For this review, take the finished solid that the model builds, in its own axes (mm). Face numbers are marked on the shaded views. A direction names the side the tool comes from. Give positions to 0.01 mm unless a question says otherwise; leave off trailing zeros. Write each loop counter-clockwise with the first axis right and the second up, starting at its lowest first coordinate (ties: lowest second). Pieces come first, ordered by that corner, then holes. Notation, with made-up numbers: (-5.5, 1.5) -> (33.5, 1.5) arc R15 cw to (33.5, 21.5) -> close; hole circle Ø4 at (63.25, 8.5). An arc over 180 degrees is marked (long way). Write item = value, one per line.
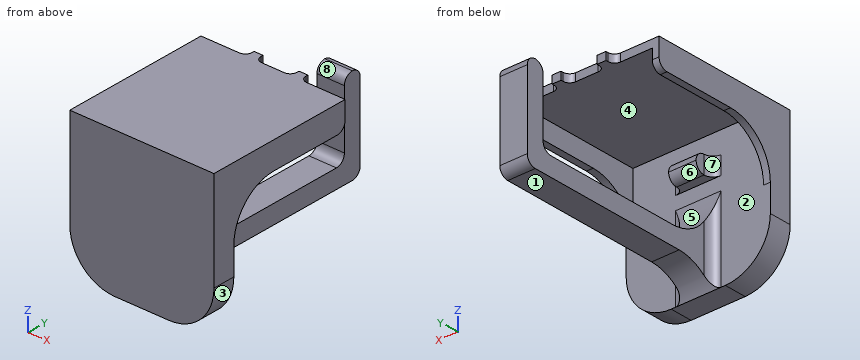
```python
from build123d import *

# Parameters (mm, degrees)
SKETCH1_W           = 32
SKETCH1_H           = 32
BOSS_EXTRUDE1_DEPTH = 5
BOSS_EXTRUDE5_DEPTH = 28
SKETCH6_W           = 6.1
SKETCH6_H           = 4.005404858
CUT_EXTRUDE2_DEPTH  = 24
SKETCH7_W           = 1.973672473
SKETCH7_H           = 2
BOSS_EXTRUDE6_DEPTH = 1.742972258
FILLET1_R           = 1.5
SKETCH8_W           = 6.1
SKETCH8_H           = 4.149014421
BOSS_EXTRUDE7_DEPTH = 42.5
SKETCH9_W           = 6.1
SKETCH9_H           = 3.972443091
BOSS_EXTRUDE8_DEPTH = 16.930897648
SKETCH10_W          = 6.1
SKETCH10_H          = 3.972443091
BOSS_EXTRUDE9_DEPTH = 4.149014421
FILLET3_R           = 2
FILLET5_R           = 10
FILLET6_R           = 2
FILLET7_R           = 10


with BuildPart() as part:
    # Sketch1 → Boss-Extrude1 (new body)
    with BuildSketch(Plane(origin=(0, 0, 0), x_dir=(1, 0, 0), z_dir=(0, 1, 0))):
        Rectangle(SKETCH1_W, SKETCH1_H)
    extrude(amount=BOSS_EXTRUDE1_DEPTH)

    # Sketch2 → Boss-Extrude5 (add)
    with BuildSketch(Plane(origin=(0, 5, 0), x_dir=(1, 0, 0), z_dir=(0, 1, 0))):
        Polygon((3.05, -5.451622884), (-3.05, -5.451622884), (-3.05, -9.457027742), (0, -9.457027742), (3.05, -9.457027742), align=None)
        Polygon((-14.5, -16), (0, -16), (14.5, -16), (16, -16), (16, -10), (14.5, -10), (14.5, -14.257027742), (0, -14.257027742), (-14.5, -14.257027742), (-14.5, -10), (-16, -10), (-16, -16), align=None)
    extrude(amount=BOSS_EXTRUDE5_DEPTH)

    # Sketch6 → Cut-Extrude2 (cut)
    with BuildSketch(Plane(origin=(0, 33, 0), x_dir=(1, 0, 0), z_dir=(0, 1, 0))):
        with Locations((0, -7.454325313)):
            Rectangle(SKETCH6_W, SKETCH6_H)
    extrude(amount=-CUT_EXTRUDE2_DEPTH, mode=Mode.SUBTRACT)

    # Sketch7 → Boss-Extrude6 (add)
    with BuildSketch(Plane.XY.offset(16)):
        with Locations((-4.986836237, 34)):
            Rectangle(SKETCH7_W, SKETCH7_H)
        with Locations((4.986836237, 34)):
            Rectangle(SKETCH7_W, SKETCH7_H)
    extrude(amount=-BOSS_EXTRUDE6_DEPTH)

    # Fillet1
    fillet1_edges = [part.edges().sort_by_distance(p)[0] for p in [
        (-5.973672473, 33, 15.128513871),
        (-4, 33, 15.128513871),
        (5.973672473, 33, 15.128513871),
        (4, 33, 15.128513871),
    ]]
    fillet(fillet1_edges, radius=FILLET1_R)

    # Sketch8 → Boss-Extrude7 (add)
    with BuildSketch(Plane(origin=(0, 5, 0), x_dir=(1, 0, 0), z_dir=(0, 1, 0))):
        with Locations((0, 9.548377117)):
            Rectangle(SKETCH8_W, SKETCH8_H)
    extrude(amount=BOSS_EXTRUDE7_DEPTH)



with BuildPart() as body_2:
    # Sketch9 → Boss-Extrude8 (new body)
    with BuildSketch(Plane.XY.offset(-7.473869906)):
        with Locations((0, 49.486221546)):
            Rectangle(SKETCH9_W, SKETCH9_H)
    extrude(amount=BOSS_EXTRUDE8_DEPTH)


with BuildPart() as part_1:
    add(part.part)

    add(body_2.part)  # Boss-Extrude9 merges body 2
    # Sketch10 → Boss-Extrude9 (add)
    with BuildSketch(Plane(origin=(0, 0, -7.473869906), x_dir=(-1, 0, 0), z_dir=(0, 0, -1))):
        with Locations((0, 49.486221546)):
            Rectangle(SKETCH10_W, SKETCH10_H)
    extrude(amount=BOSS_EXTRUDE9_DEPTH)

    # Fillet3
    # the kernel refuses this fillet: 2 mm, written as the material it adds along each edge
    with BuildSketch(Plane(origin=(3.05, 47.5, -7.473869906), x_dir=(0, 0, 1), z_dir=(-1, 0, 0))) as fillet3_piece_1:
        with BuildLine():
            CenterArc((FILLET3_R, -FILLET3_R), FILLET3_R, 90, 90)
            Line((0, -FILLET3_R), (0, 0))
            Line((0, 0), (FILLET3_R, 0))
        make_face()
    extrude(amount=6.1)
    # the kernel refuses this fillet: 2 mm, written as the material it takes off along each edge
    with BuildSketch(Plane(origin=(8.05, 51.472443091, -11.622884327), x_dir=(0, -1, 0), z_dir=(-1, 0, 0)), Plane(origin=(-8.05, 51.472443091, 9.457027742), x_dir=(0, -1, 0), z_dir=(1, 0, 0))) as fillet3_2_piece_1:
        with BuildLine():
            CenterArc((FILLET3_R, FILLET3_R), FILLET3_R, 180, 90)
            Line((0, FILLET3_R), (0, 0))
            Line((0, 0), (FILLET3_R, 0))
        make_face()
    extrude(amount=16.1, mode=Mode.SUBTRACT)
    with BuildSketch(Plane(origin=(8.05, 47.5, 9.457027742), x_dir=(0, 0, -1), z_dir=(-1, 0, 0)), Plane(origin=(-8.05, 9, 5.451622884), x_dir=(0, -1, 0), z_dir=(1, 0, 0)), Plane(origin=(8.05, 9, 9.457027742), x_dir=(0, -1, 0), z_dir=(-1, 0, 0))) as fillet3_2_piece_2:
        with BuildLine():
            CenterArc((FILLET3_R, -FILLET3_R), FILLET3_R, 90, 90)
            Line((0, -FILLET3_R), (0, 0))
            Line((0, 0), (FILLET3_R, 0))
        make_face()
    extrude(amount=16.1, mode=Mode.SUBTRACT)
    with BuildSketch(Plane(origin=(21, 33, 10), x_dir=(0, 0, 1), z_dir=(-1, 0, 0)), Plane(origin=(-9.5, 33, 10), x_dir=(0, 0, 1), z_dir=(-1, 0, 0))) as fillet3_2_piece_3:
        with BuildLine():
            CenterArc((FILLET3_R, -FILLET3_R), FILLET3_R, 90, 90)
            Line((0, -FILLET3_R), (0, 0))
            Line((0, 0), (FILLET3_R, 0))
        make_face()
    extrude(amount=11.5, mode=Mode.SUBTRACT)

    # Fillet5
    # the kernel refuses this fillet: 10 mm, written as the material it adds along each edge
    with BuildSketch(Plane(origin=(-3.05, 5, -7.473869906), x_dir=(0, 1, 0), z_dir=(1, 0, 0))) as fillet5_piece_1:
        with BuildLine():
            CenterArc((FILLET5_R, FILLET5_R), FILLET5_R, 180, 90)
            Line((0, FILLET5_R), (-FILLET5_R * 0.02, FILLET5_R))
            Line((-FILLET5_R * 0.02, FILLET5_R), (-FILLET5_R * 0.02, -FILLET5_R * 0.02))
            Line((-FILLET5_R * 0.02, -FILLET5_R * 0.02), (FILLET5_R, -FILLET5_R * 0.02))
            Line((FILLET5_R, -FILLET5_R * 0.02), (FILLET5_R, 0))
        make_face()
    extrude(amount=6.1)
    with BuildSketch(Plane(origin=(3.05, 5, -11.622884327), x_dir=(0, 0, -1), z_dir=(-1, 0, 0))) as fillet5_piece_2:
        with BuildLine():
            CenterArc((10, -8.26941182), FILLET5_R, 124.214206314, 55.785793686)
            Line((0, -8.26941182), (-0.2, -8.26941182))
            Line((-0.2, -8.26941182), (-0.2, 0))
            Line((-0.2, 0), (0, 0.2))
            ThreePointArc((0, 0.2), (2.188557837, 0.2), (4.264657987, 0.165388236))
            Line((4.264657987, 0.165388236), (4.377115673, 0))
        make_face()
    extrude(amount=6.1)
    with BuildSketch(Plane(origin=(-14.5, 5, 10), x_dir=(0, 0, -1), z_dir=(-1, 0, 0)), Plane(origin=(16, 5, 10), x_dir=(0, 0, -1), z_dir=(-1, 0, 0))) as fillet5_piece_3:
        with BuildLine():
            CenterArc((FILLET5_R, -FILLET5_R), FILLET5_R, 90, 90)
            Line((0, -FILLET5_R), (-FILLET5_R * 0.02, -FILLET5_R))
            Line((-FILLET5_R * 0.02, -FILLET5_R), (-FILLET5_R * 0.02, FILLET5_R * 0.02))
            Line((-FILLET5_R * 0.02, FILLET5_R * 0.02), (FILLET5_R, FILLET5_R * 0.02))
            Line((FILLET5_R, FILLET5_R * 0.02), (FILLET5_R, 0))
        make_face()
    extrude(amount=1.5)

    # Fillet6
    fillet6_edges = [part_1.edges().sort_by_distance(p)[0] for p in [
        (-3.05, 5, -6.736934953),
        (-3.05, 5, 7.454325313),
        (3.05, 5, -6.736934953),
        (3.05, 5, 7.454325313),
    ]]
    fillet(fillet6_edges, radius=FILLET6_R)

    # Fillet7
    fillet7_edges = [part_1.edges().sort_by_distance(p)[0] for p in [
        (-16, 2.5, -16),
        (16, 2.5, -16),
    ]]
    fillet(fillet7_edges, radius=FILLET7_R)


solid = part_1.part
```
(1) For pin 1 (1.9 mm diameter, centred on x = -0.5, z = 15.5, fed in from +Y); pin 2 (5 mm diameter, centred on x = -9.5, y = 33, fed in from -Z); pin 3 (0.5 mm diameter, centred on x = -5, z = 15.5, fed in from +Y), all flat-tipped, find the tip position at first contact; note any pin that passes through.
Answers below:
pin_1 = 33
pin_2 = 14.26
pin_3 = 35
(2) The part is to be moulded in two halves that separate along X. For the marked faces 1, 2 and 3, say which applies: released by +X, released by -X, zero draft, split by the parting line, or undercut.
Answers below:
face_1 = zero draft
face_2 = undercut
face_3 = released by +X
(3) Take a section at A-A (y = 29). Write out the cut boundary in (x, z), plus the area to 3 significant figures.
Answers below:
outline = (-16, 10) -> (-14.5, 10) -> (-14.5, 14.26) -> (14.5, 14.26) -> (14.5, 10) -> (16, 10) -> (16, 16) -> (-16, 16) -> close; (-3.05, -11.62) -> (3.05, -11.62) -> (3.05, -7.47) -> (-3.05, -7.47) -> close
area = 93.9 mm^2
(4) Tool access review of the marked faces 4, 5, 6, 7 and 8: name each direction out of +Z, -Z, +X, -X, +Y, -Y from which nothing blocks a thin tool from reaching the whole face with its end or side.
Answers below:
face_4 = +Y
face_5 = none
face_6 = +X, -X
face_7 = -Z, +Y
face_8 = +Z, +X, -X
(5) To check wall thickness, follow probe 1 along X at (y, z) = (8, 12); probe 2 along Z at (x, y) = (13, 7). State the ranges of each line that lie inside material, in increasing order.
Answers below:
probe_1 = -16 to -14.5, 14.5 to 16
probe_2 = 14.26 to 16
